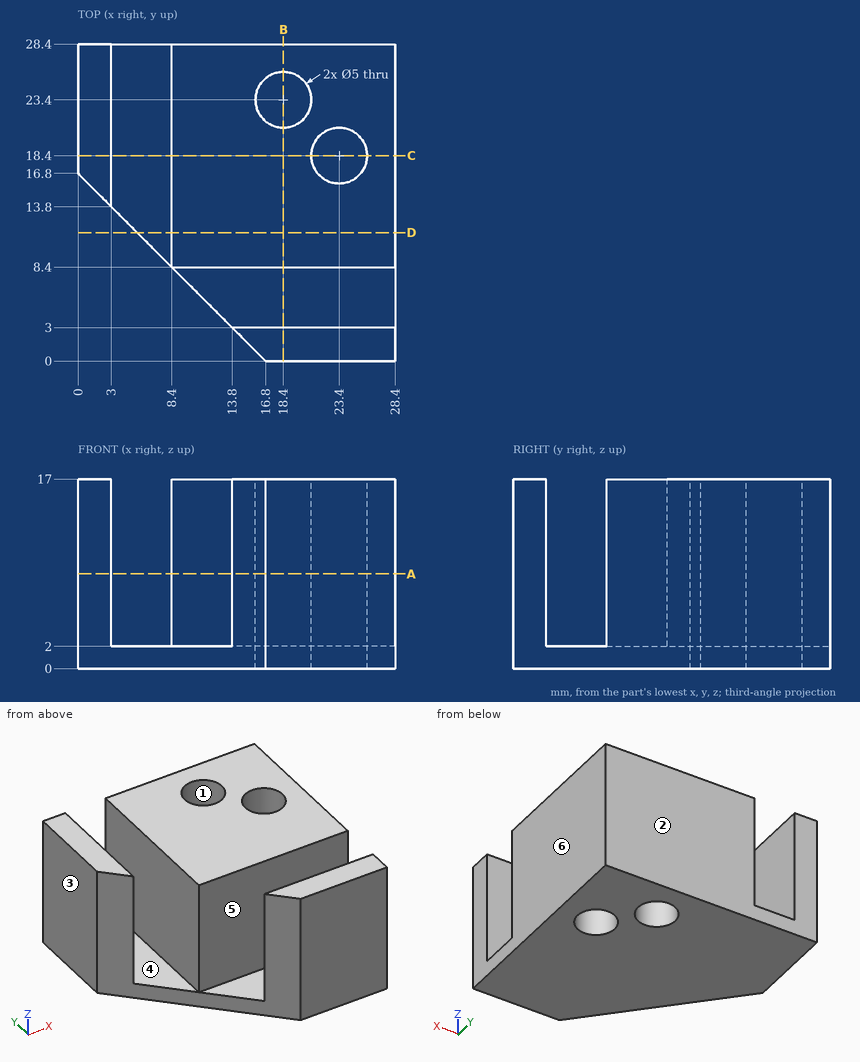
Design review of the part shown in the three views and the two pictorial views. Dimensions are in mm from the part's minimum x, y and z. A direction names the side the tool comes from. Coordinates: 2 decimals unless noted, no trailing zeros. Loops run counter-clockwise (first coordinate to the right, second up) from the corner with the lowest first, then second, coordinate; pieces in that order, holes last.
Q1. The part is to be moulded in two halves that separate along Y. For the marked faces 1, 2 and 3, say which applies: +Y half, -Y half, draft (parallel to the pull), parting line (faces both ways), or undercut.
Reported:
face 1: undercut
face 2: +Y half
face 3: draft
Q2. To check wall thickness, follow line 1 (Y direction, x = 18.4, z = 5.75); line 2 (Y direction, x = 23.4, z = 12.5). State the ranges of each line that lie inside material, in increasing order.
Reported:
line 1: y = 0 to 3, 8.4 to 20.9, 25.9 to 28.4
line 2: y = 0 to 3, 8.4 to 15.9, 20.9 to 28.4
Q3. We need section A-A on z = 8.5. State the section outline as (x, y) points, and give its area (3 significant figures).
Reported:
outline: (0, 16.8) - (3, 13.8) - (3, 28.4) - (0, 28.4) - close; (8.4, 8.4) - (28.4, 8.4) - (28.4, 28.4) - (8.4, 28.4) - close; (13.8, 3) - (16.8, 0) - (28.4, 0) - (28.4, 3) - close; hole circle Ø5 at (18.4, 23.4); hole circle Ø5 at (23.4, 18.4)
area: 439 mm2
Q4. Tool access review of the marked faces 4, 5 and 6: name each direction out of +Z, -Z, +X, -X, +Y, -Y from which nothing blocks a thin tool from reaching the whole face with its end or side.
Reported:
face 4: +Z, +Y, -Y
face 5: +Z, +X, -X
face 6: +Z, -Z, +X, +Y, -Y
Q5. For pin 1 (5 mm diameter, centred on y = 7.5, z = 15.5, fed in from +X); pin 2 (3 mm diameter, centred on x = 10.5, y = 4, fed in from +Z), all flat-tipped, find the tip position at first contact; note any pin that passes through.
Reported:
pin 1: stops at x = 28.4
pin 2: passes through
Q6. We need section D-D on y = 11.5. State the section outline as (x, z) points, and give its area (3 significant figures).
Reported:
outline: (5.3, 0) - (28.4, 0) - (28.4, 17) - (8.4, 17) - (8.4, 2) - (5.3, 2) - close
area: 346 mm2
Q7. We need section B-B on x = 18.4. State the section outline as (y, z) points.
Reported:
outline: (0, 0) - (20.9, 0) - (20.9, 17) - (8.4, 17) - (8.4, 2) - (3, 2) - (3, 17) - (0, 17) - close; (25.9, 0) - (28.4, 0) - (28.4, 17) - (25.9, 17) - close
